Autodesk Inventor part; units mm, degrees
ref_plane "YZ Plane" through (0, 0, 0) normal (1, 0, 0) x (0, 1, 0)
ref_plane "XZ Plane" through (0, 0, 0) normal (0, 1, 0) x (-1, 0, 0)
ref_plane "XY Plane" through (0, 0, 0) normal (0, 0, 1) x (1, 0, 0)
sketch "Sketch1" plane through (0, 0, 0) normal (1, 0, 0) x (0, 1, 0)
  line L0 (0, 0) -> (25.4, 0)
  line L1 (25.4, 0) -> (25.4, -38.1)
  line L2 (25.4, -38.1) -> (0, -38.1)
  line L3 (0, -38.1) -> (0, 0)
  line L4 (25.4, 0) -> (25.4, -6.35)
  line L5 (25.4, -6.35) -> (19.05, -6.35)
  line L6 (19.05, -6.35) -> (6.35, -6.35)
  circle A0 centre (19.05, -6.35) radius 2.1082
  circle A1 centre (6.35, -6.35) radius 2.1082
  dimension "d0" = 38.1
  dimension "d1" = 25.4
  dimension "d2" = 6.35
  dimension "d3" = 6.35
  dimension "d4" = 12.7
  dimension "d5" = 4.2164
extrude "Extrusion1" add sketch "Sketch1" along normal blind 12.7
sketch "Sketch2" plane through (0, 25.4, 0) normal (0, 1, 0) x (1, 0, 0)
  line L0 (0, 0) -> (0, 38.1)
  line L1 (0, 38.1) -> (12.7, 38.1)
  line L2 (0, 38.1) -> (12.7, 38.1)
  circle A0 centre (6.35, 12.7) radius 2.1082
  line L3 (0, 0) -> (12.7, 0)
  line L4 (6.35, 0) -> (6.35, 12.7)
  dimension "d9" = 4.2164
extrude "Extrusion2" cut sketch "Sketch2" against normal blind 39.6875
fillet "Fillet1" radius 3.175 8 edges at (12.7, 12.7, 0) (12.7, 25.4, -19.05) (6.35, 25.4, -38.1) (12.7, 12.7, -38.1) (12.7, 0, -19.05) (6.35, 25.4, 0) (6.35, 0, 0) (6.35, 0, -38.1)
sketch "Sketch5" plane through (0, 25.4, -3.175) normal (0, 1, 0) x (1, 0, 0)
  circle A0 centre (6.35, 9.525) radius 2.1082
  line L0 (6.35, 9.525) -> (6.35, 23.495)
  line L1 (6.35, 23.495) -> (5.334, 23.495)
  circle A1 centre (5.334, 23.495) radius 2.1082
  point P0 (0, -3.175)
  dimension "d22" = 13.97
  dimension "d23" = 1.016
  dimension "d24" = 4.2164
extrude "Extrusion5" cut sketch "Sketch5" against normal blind 57.15 contours A1
sketch "Sketch6" plane through (0, 0, 0) normal (-1, 0, 0) x (0, 0, 1)
  circle A0 centre (-6.35, 6.35) radius 2.1082
  line L0 (-6.35, 6.35) -> (-50.8, 6.35)
  circle A1 centre (-50.8, 6.35) radius 2.1082
  line L1 (-3.175, 0) -> (-34.925, 0)
  line L2 (-3.175, 25.4) -> (-3.175, 22.225)
  line L3 (-3.175, 0) -> (-3.175, 25.4)
  line L4 (-3.175, 0) -> (-60.325, 0)
  line L5 (-60.325, 0) -> (-60.325, 12.7)
  line L6 (-60.325, 12.7) -> (-3.175, 12.7)
  line L7 (-3.175, 12.7) -> (-3.175, 0)
  line L8 (-34.925, 0) -> (-34.925, 12.7)
  line L9 (-34.925, 22.225) -> (-34.925, 3.175)
  point P0 (0, 0)
  point P1 (-34.925, 0)
  dimension "d27" = 44.45
  dimension "d28" = 57.15
extrude "Extrusion6" add sketch "Sketch6" against normal blind 6.35 contours L4 L5 L6 L8
fillet "Fillet2" radius 3.175 2 edges at (3.175, 12.7, -60.325) (3.175, 0, -60.325)
properties part number "wing mount 1 v1"
Input: part model. Units: mm. Frame: model coordinates. A direction names the side the tool comes from. Give positions to 0.01 mm unless a question says otherwise; leave off trailing zeros. Loops run counter-clockwise (first coordinate to the right, second up) from the corner with the lowest first, then second, coordinate; pieces in that order, holes last. Notation, with made-up numbers: (-39.75, 84.25) -> (-11.75, 84.25) arc R25 cw to (-11.75, 110.25) -> close; hole circle Ø9 at (36.25, -16.5). An arc over 180 degrees is marked (long way). Answer as a JSON object with one key per item and string values. Group by question number.
Item 1: Pin query (flat end, axial travel): P1, Ø4, axis at x = 6, y = 12.5, coming from the -Z side; P2, Ø5, axis at x = 5.334, z = -26.67, coming from the -Y side; P3, Ø1.5, axis at x = 9, y = 3.5, coming from the -Z side; P4, Ø14, axis at y = 3.5, z = -52.5, coming from the +X side. Return the tip coordinate at first contact, or that it passes through.
Item 2: Reachability of faces 5 (the flat face through (0, 13, -24)), 6 (the flat face through (3, 12.7, -48)), 7 (the cylindrical face through (7.96, 0.91, -37.15)) from +Z, -Z, +X, -X, +Y, -Y: full face, straight path, thin tool, end or side. Return the list, or none.
Item 3: Pull-direction query (X, two-part tool) for faces 1 (the cylindrical face through (4.83, 0.95, -0.91)), 2 (the cylindrical face through (11.75, 12.83, -0.91)), 3 (the cylindrical face through (3.66, 12.88, -25.39)), 4 (the cylindrical face through (6.08, 12.88, -14.79)); classes: released by +X, released by -X, zero draft, split by the parting line, or undercut.
Item 4: Cut plane B-B, the plane x = 5.5. Return the cut outline in (y, z) (3 decimals).
Item 5: Cut plane D-D, the plane y = 5. Return the cut outline in (x, z) (3 decimals), and give its area (3 significant figures).
Item 6: Cut plane C-C, the plane z = -50.8. Return the cut outline in (x, y), and give its area (3 significant figures).
Item 7: Line query: probe 1 along Y at (x, z) = (2.25, -50.8); probe 2 along Z at (x, y) = (6, 12). Output: solid intervals per line, ascending.
Item 8: Cut plane A-A, the plane y = 19.05. Return the cut outline in (x, z) (3 decimals).
Checks:
{
 "1": {"P1": "stops at z = -60.17", "P2": "stops at y = 0", "P3": "stops at z = -38.1", "P4": "stops at x = 6.35"},
 "2": {"face 5": "+Z, -Z, -X, +Y, -Y", "face 6": "-Z, +X, -X, +Y", "face 7": "-Z, +X, -Y"},
 "3": {"face 1": "zero draft", "face 2": "released by +X", "face 3": "undercut", "face 4": "undercut"},
 "4": {"outline": "(0, -57.15) arc R3.175 ccw to (3.175, -60.325) -> (9.525, -60.325) arc R3.175 ccw to (12.7, -57.15) -> (12.7, -38.1) -> (22.225, -38.1) arc R3.175 ccw to (25.4, -34.925) -> (25.4, -28.772) -> (0, -28.772) -> close; (0, -24.568) -> (25.4, -24.568) -> (25.4, -14.629) -> (0, -14.629) -> close; (0, -10.771) -> (25.4, -10.771) -> (25.4, -3.175) arc R3.175 ccw to (22.225, 0) -> (3.175, 0) arc R3.175 ccw to (0, -3.175) -> close; hole circle Ø4.216 at (6.35, -50.8); hole circle Ø4.216 at (6.35, -6.35); hole circle Ø4.216 at (19.05, -6.35)"},
 "5": {"outline": "(0, -60.325) -> (6.35, -60.325) -> (6.35, -52.419) -> (0, -52.419) -> close; (0, -49.181) -> (6.35, -49.181) -> (6.35, -38.1) -> (9.525, -38.1) arc R3.175 ccw to (12.7, -34.925) -> (12.7, -7.969) -> (0, -7.969) -> close; (0, -4.731) -> (12.7, -4.731) -> (12.7, -3.175) arc R3.175 ccw to (9.525, 0) -> (0, 0) -> close; hole circle Ø4.216 at (5.334, -26.67); hole circle Ø4.216 at (6.35, -12.7)", "area": "531 mm²"},
 "6": {"outline": "(0, 0) -> (6.35, 0) -> (6.35, 4.24) -> (0, 4.24) -> close; (0, 8.46) -> (6.35, 8.46) -> (6.35, 12.7) -> (0, 12.7) -> close", "area": "53.9 mm²"},
 "7": {"probe 1": "y = 0 to 4.24, 8.46 to 12.7", "probe 2": "z = -59.14 to -28.67, -24.67 to -14.78, -10.62 to 0"},
 "8": {"outline": "(0, -38.1) -> (9.525, -38.1) arc R3.175 ccw to (12.7, -34.925) -> (12.7, -8.458) -> (0, -8.458) -> close; (0, -4.242) -> (12.7, -4.242) -> (12.7, -3.175) arc R3.175 ccw to (9.525, 0) -> (0, 0) -> close; hole circle Ø4.216 at (5.334, -26.67); hole circle Ø4.216 at (6.35, -12.7)"}
}
